Work out the finished part from the listing and answer in its coordinate system (mm). Coordinates: 2 decimals unless noted, no trailing zeros. Order: outer loops, then holes, each group sorted by start corner. A loop starts at its lowest first (then second) coordinate and runs counter-clockwise, first axis right, second up. Notation, with made-up numbers: (85.5, 54.25) - (122.5, 54.25) arc R21 cw to (122.5, 90.25) - close; hole circle Ø5 at (42, 77.25). An arc over 180 degrees is marked (long way). Use CSV: the item, a comma, the result in double quotes. Start each with the question number.
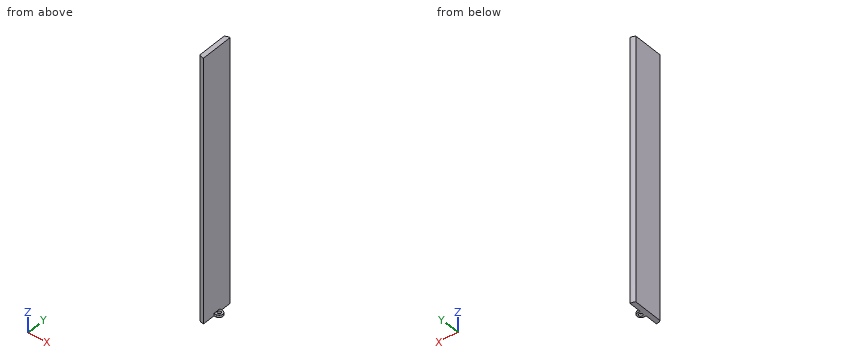
from build123d import *

# Parameters (mm, degrees)
EXTRUDE_1_DEPTH = 110
SKETCH_1_4_R    = 0.75
EXTRUDE_2_DEPTH = 1


with BuildPart() as part:
    # Sketch 1 → Extrude 1 (new body)
    with BuildSketch(Plane.XY):
        with BuildLine():
            Line((-1, 6.92820323), (-1, 1.5))
            Line((-1, 1.5), (-1, -1.5))
            Line((-1, -1.5), (-1, -6.92820323))
            ThreePointArc((-1, -6.92820323), (-2.022646212, -6.701410471), (-3, -6.32455532))
            Line((-3, -6.32455532), (-3, 6.32455532))
            ThreePointArc((-3, 6.32455532), (-2.022646212, 6.701410471), (-1, 6.92820323))
        make_face()
    extrude(amount=EXTRUDE_1_DEPTH)

    # Sketch 1_4 → Extrude 2 (add)
    with BuildSketch(Plane.XY):
        with BuildLine():
            Line((0, -1.5), (-1, -1.5))
            Line((-1, -1.5), (-1, 1.5))
            Line((-1, 1.5), (0, 1.5))
            ThreePointArc((0, 1.5), (1.5, 0), (0, -1.5))
        make_face()
        Circle(SKETCH_1_4_R, mode=Mode.SUBTRACT)
    extrude(amount=EXTRUDE_2_DEPTH)


solid = part.part
1) Straight lines are drawn through the part: line 1 (Y direction, x = 0, z = 0.5); line 2 (X direction, y = -1, z = 24.5); line 3 (Z direction, x = 0.2, y = 1). For each, find the intervals that lie inside material, in ascending order. Write a range as [from, to].
2) The part is cut by section B-B on z = 58. Determine the outline of the cut face in (x, y), plus the area to 3 significant figures.
3) Flat-ended cylindrical pins translate along their axes: P1, Ø4, axis at y = 4, z = 64.5, coming from the +X side; P2, Ø2, axis at x = 0.5, z = 53.5, coming from the +Y side; P3, Ø0.5, axis at x = -0.5, z = 0.5, coming from the +Y side; P4, Ø2, axis at x = -2.5, z = 97.5, coming from the -Y side. Find the tip coordinate at first contact, or state that the pin passes through.
4) The part is cut by section A-A on y = 5. Determine the outline of the cut face in (x, z).
Answer key:
1,line 1,"[-1.5, -0.75], [0.75, 1.5]"
1,line 2,"[-3, -1]"
1,line 3,"[0, 1]"
2,outline,"(-3, -6.32) arc R7 ccw to (-1, -6.93) - (-1, 6.93) arc R7 ccw to (-3, 6.32) - close"
2,area,"26.7 mm^2"
3,P1,"x = -1"
3,P2,"through"
3,P3,"y = 1.5"
3,P4,"y = -6.84"
4,outline,"(-3, 0) - (-1, 0) - (-1, 110) - (-3, 110) - close"
